Build history of the part. All positions in model axes, mm. Face numbers are marked on the shaded views. A direction names the side the tool comes from. Round coordinates to 2 decimals unless told otherwise and drop trailing zeros. Order: outer loops, then holes, each group sorted by start corner. A loop starts at its lowest first (then second) coordinate and runs counter-clockwise, first axis right, second up. Notation, with made-up numbers: M 30,63 L 38,63 A12 ccw 38,75 Z; hole C -28.5,16.25 d3. An arc over 180 degrees is marked long. One line per item, written item: value. Start each with the question number.
Item 1: Band-saw the part on B-B, the plane x = 128.25. Write the cut outline in (y, z).
Item 2: Tool access for the marked faces 1, 2, 3 and 4: list every direction of +Z, -Z, +X, -X, +Y, -Y with a clear straight run to the whole face (end or side of a thin tool).
Item 3: Probe L1, parallel to Y at x = 128.25, z = -9.5; L2, parallel to Z at x = 64, y = 2; L3, parallel to X at y = 4.75, z = -9.25. List the from-to ranges inside material, lowest first.
Item 4: Two-plate mould, pull along X, no slides. Class the marked faces 5, 6 and 7: +X half, -X half, draft (parallel to the pull), parting line (faces both ways), or undercut.
Item 5: Band-saw the part on A-A, the plane x = 59.5. Write the cut outline in (y, z), then the cut area to 3 significant figures.
Item 6: Pin check, flat tips, straight feed: pin 1 (3 mm diameter, centred on x = 109, z = -17.5, fed in from +Y); pin 2 (8 mm diameter, centred on x = 127.5, y = 2, fed in from -Z); pin 3 (6 mm diameter, centred on y = -2, z = -3.5, fed in from +X). Stop position of each tip, or through.
```python
from build123d import *

# Parameters (mm, degrees)
SKETCH1_W           = 150
SKETCH1_H           = 20
SKETCH1_R           = 0.9
BOSS_EXTRUDE1_DEPTH = 5
SKETCH2_R           = 1.95
CUT_EXTRUDE1_DEPTH  = 2.9
SKETCH3_W           = 55.59541546
SKETCH3_H           = 20
BOSS_EXTRUDE2_DEPTH = 5
SKETCH7_W           = 20
SKETCH7_H           = 5
CUT_EXTRUDE3_DEPTH  = 27.6
SKETCH5_R           = 1.25
CUT_EXTRUDE4_DEPTH  = 27.6
SKETCH8_W           = 7.5
SKETCH8_H           = 20
BOSS_EXTRUDE3_DEPTH = 5
SKETCH9_R           = 1.25
CUT_EXTRUDE5_DEPTH  = 43
CHAMFER2_SIZE       = 2
CHAMFER3_SIZE       = 2
CHAMFER4_SIZE       = 5
SKETCH12_W          = 65.05458454
SKETCH12_H          = 15
SKETCH12_W_2        = 27.005472272
CUT_EXTRUDE33_DEPTH = 43
FILLET3_R           = 5
CHAMFER5_SIZE       = 5
CUT_EXTRUDE35_DEPTH = 34
SKETCH14_W          = 15
SKETCH14_H          = 5
BOSS_EXTRUDE4_DEPTH = 6
BOSS_EXTRUDE5_DEPTH = 18
CHAMFER7_SIZE       = 2
BOSS_EXTRUDE6_DEPTH = 1
CHAMFER8_SIZE       = 5


with BuildPart() as part:
    # Sketch1 → Boss-Extrude1 (new body)
    with BuildSketch(Plane(origin=(0, 0, 0), x_dir=(1, 0, 0), z_dir=(0, 1, 0))):
        with Locations((75, 10)):
            Rectangle(SKETCH1_W, SKETCH1_H)
        with Locations(Location((40, 10, 0), (0, 0, 270))):
            Circle(SKETCH1_R, mode=Mode.SUBTRACT)
    extrude(amount=BOSS_EXTRUDE1_DEPTH)

    # Sketch2 → Cut-Extrude1 (cut)
    with BuildSketch(Plane.XZ):
        with Locations(Location((40, -10, 0), (0, 0, 270))):
            Circle(SKETCH2_R)
    extrude(amount=-CUT_EXTRUDE1_DEPTH, mode=Mode.SUBTRACT)

    # Sketch3 → Boss-Extrude2 (add)
    with BuildSketch(Plane.XZ):
        with Locations((122.20229227, -10)):
            Rectangle(SKETCH3_W, SKETCH3_H)
    extrude(amount=BOSS_EXTRUDE2_DEPTH)

    # Sketch7 → Cut-Extrude3 (cut)
    with BuildSketch(Plane.ZY.offset(-94.40458454)):
        with Locations((-10, -2.5)):
            Rectangle(SKETCH7_W, SKETCH7_H)
    extrude(amount=-CUT_EXTRUDE3_DEPTH, mode=Mode.SUBTRACT)

    # Sketch5 → Cut-Extrude4 (cut)
    with BuildSketch(Plane(origin=(0, 0, -20), x_dir=(-1, 0, 0), z_dir=(0, 0, -1))):
        with Locations((-128.25, 0)):
            Circle(SKETCH5_R)
        with Locations((-143.75, 0)):
            Circle(SKETCH5_R)
    extrude(amount=-CUT_EXTRUDE4_DEPTH, mode=Mode.SUBTRACT)

    # Sketch8 → Boss-Extrude3 (add)
    with BuildSketch(Plane(origin=(0, 5, 0), x_dir=(1, 0, 0), z_dir=(0, 1, 0))):
        with Locations((3.75, 10)):
            Rectangle(SKETCH8_W, SKETCH8_H)
    extrude(amount=BOSS_EXTRUDE3_DEPTH)

    # Sketch9 → Cut-Extrude5 (cut)
    with BuildSketch(Plane(origin=(0, 0, -20), x_dir=(-1, 0, 0), z_dir=(0, 0, -1))):
        with Locations((-3.75, 5)):
            Circle(SKETCH9_R)
    extrude(amount=-CUT_EXTRUDE5_DEPTH, mode=Mode.SUBTRACT)

    # Chamfer2
    chamfer2_edges = [part.edges().sort_by_distance(p)[0] for p in [
        (7.5, 5, -10),
    ]]
    chamfer(chamfer2_edges, length=CHAMFER2_SIZE)

    # Chamfer3
    chamfer3_edges = [part.edges().sort_by_distance(p)[0] for p in [
        (0, 0, -10),
    ]]
    chamfer(chamfer3_edges, length=CHAMFER3_SIZE)

    # Chamfer4
    chamfer4_edges = [part.edges().sort_by_distance(p)[0] for p in [
        (122.00458454, 0, -10),
    ]]
    chamfer(chamfer4_edges, length=CHAMFER4_SIZE - 0.0001)  # a hair under: the kernel refuses the full size

    # Sketch12 → Cut-Extrude33 (cut)
    with BuildSketch(Plane.XZ):
        with Locations((79.47729227, -10)):
            Rectangle(SKETCH12_W, SKETCH12_H)
        with Locations((19.547263864, -10)):
            Rectangle(SKETCH12_W_2, SKETCH12_H)
    extrude(amount=-CUT_EXTRUDE33_DEPTH, mode=Mode.SUBTRACT)

    # Fillet3
    fillet3_edges = [part.edges().sort_by_distance(p)[0] for p in [
        (6.044527728, 5, -17.5),
        (6.044527728, 5, -2.5),
    ]]
    fillet(fillet3_edges, radius=FILLET3_R)

    # Chamfer5
    chamfer5_edges = [part.edges().sort_by_distance(p)[0] for p in [
        (46.95, 2.5, -17.5),
        (46.95, 2.5, -2.5),
        (33.05, 2.5, -2.5),
        (33.05, 2.5, -17.5),
    ]]
    chamfer(chamfer5_edges, length=CHAMFER5_SIZE)

    # Sketch13 → Cut-Extrude35 (cut)
    with BuildSketch(Plane(origin=(150, 0, 0), x_dir=(0, 0, -1), z_dir=(1, 0, 0))):
        Polygon((5, 5), (0, 5), (0, -5), (5, -5), (7.5, -5), (7.5, 5), align=None)
        Polygon((15, 5), (12.5, 5), (12.5, -5), (15, -5), (20, -5), (20, 5), align=None)
    extrude(amount=-CUT_EXTRUDE35_DEPTH, mode=Mode.SUBTRACT)

    # Sketch14 → Boss-Extrude4 (add)
    with BuildSketch(Plane.ZY.offset(-112.00458454)):
        with Locations((-10, 2.5)):
            Rectangle(SKETCH14_W, SKETCH14_H)
    extrude(amount=BOSS_EXTRUDE4_DEPTH)

    # Sketch15 → Boss-Extrude5 (add)
    with BuildSketch(Plane.ZY.offset(-106.00458454)):
        Polygon((-10, 5), (-7.5, 5), (-7.5, -5), (-12.5, -5), (-12.5, 5), align=None)
    extrude(amount=-BOSS_EXTRUDE5_DEPTH)

    # Chamfer7
    chamfer7_edges = [part.edges().sort_by_distance(p)[0] for p in [
        (106.00458454, -5, -10),
        (111.00229227, 0, -7.5),
        (111.00229227, 0, -12.5),
    ]]
    chamfer(chamfer7_edges, length=CHAMFER7_SIZE)

    # Sketch17 → Boss-Extrude6 (add)
    with BuildSketch(Plane(origin=(116, 0, 0), x_dir=(0, 0, -1), z_dir=(1, 0, 0))):
        Polygon((0, 0), (5.5, 0), (7.5, -2), (7.5, 5), (0, 5), align=None)
        Polygon((12.5, 5), (12.5, -2), (14.5, 0), (20, 0), (20, 5), align=None)
    extrude(amount=BOSS_EXTRUDE6_DEPTH)

    # Chamfer8
    chamfer8_edges = [part.edges().sort_by_distance(p)[0] for p in [
        (117, 1.5, -12.5),
        (117, 1.5, -7.5),
    ]]
    chamfer(chamfer8_edges, length=CHAMFER8_SIZE)


solid = part.part
```
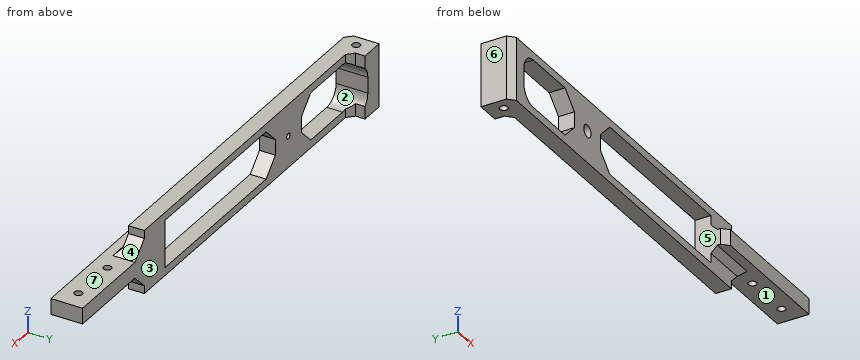
Output:
1. outline: M -5,-12.5 L -1.25,-12.5 L -1.25,-7.5 L -5,-7.5 Z; M 1.25,-12.5 L 5,-12.5 L 5,-7.5 L 1.25,-7.5 Z
2. face 1: -Z, +X, -Y
2. face 2: +Y, -Y
2. face 3: +Z, -Z, +X, +Y
2. face 4: +Z, +X, +Y, -Y
3. L1: y = -5 to -1.25, 1.25 to 5
3. L2: z = -20 to -17.5, -2.5 to 0
3. L3: x = 0 to 2.53, 4.97 to 6.04, 33.05 to 39.5, 40.5 to 46.95, 106 to 150
4. face 5: undercut
4. face 6: -X half
4. face 7: draft
5. outline: M 0,-20 L 5,-20 L 5,-17.5 L 0,-17.5 Z; M 0,-2.5 L 5,-2.5 L 5,0 L 0,0 Z
5. area: 25.0 mm²
6. pin 1: stops at y = 5
6. pin 2: stops at z = -12.5
6. pin 3: stops at x = 120.71
